Geometry: final body of the model. Coordinates: model frame, mm. A direction names the side the tool comes from. Round coordinates to 2 decimals unless told otherwise and drop trailing zeros. Loops run counter-clockwise (first coordinate to the right, second up) from the corner with the lowest first, then second, coordinate; pieces in that order, holes last. Notation, with made-up numbers: (-32.75, -6.75) - (-2.75, -6.75) arc R17 cw to (-2.75, -2.75) - close; hole circle Ø9 at (26, -14.75). An arc over 180 degrees is marked (long way). Answer in a Markdown table with one row per item. Add a question column.
from build123d import *

# Parameters (mm, degrees)
F0_R      = 18
F1_DEPTH  = 25
F2_R      = 6.5
F3_DEPTH  = 4.5
F4_R      = 1.5875
F5_DEPTH  = 9
F6_W      = 1
F6_H      = 2
F7_DEPTH  = 4.5
F8_R      = 1.5
F9_DEPTH  = 5
F10_R     = 2.5
F11_DEPTH = 4.5


# Not quite as in the source:
# - a pattern or mirror of a feature is missing from the dataset's text; its kind, count and spacing are read off the source's solid


with BuildPart() as f1:
    # F0 (on Top) → F1 (new body, symmetric)
    with BuildSketch(Plane.XY):
        Circle(F0_R)
    extrude(amount=F1_DEPTH, both=True)

    # F2 (on face) → F3 (join)
    with BuildSketch(Plane.XY.offset(25)):
        Circle(F2_R)
    extrude(amount=F3_DEPTH)

    # F4 (on face) → F5 (join)
    with BuildSketch(Plane.XY.offset(29.5)):
        Circle(F4_R)
    extrude(amount=F5_DEPTH)

    # F6 (on face) → F7 (join)
    with BuildSketch(Plane(origin=(0, 0, -25), x_dir=(1, 0, 0), z_dir=(0, 0, -1))):
        with Locations((-14.5, 0)):
            Rectangle(F6_W, F6_H)
    f7 = extrude(amount=F7_DEPTH)

    # F7_copies: F7 across plane
    add(f7.mirror(Plane(origin=(0, 0, 0), x_dir=(0, 0, 1), z_dir=(1, 0, 0))))

    # F8 (on face) → F9 (cut)
    with BuildSketch(Plane.XY.offset(25)):
        with Locations((12.5, 0)):
            Circle(F8_R)
        with Locations((-12.5, 0)):
            Circle(F8_R)
    extrude(amount=-F9_DEPTH, mode=Mode.SUBTRACT)

    # F10 (on face) → F11 (join)
    with BuildSketch(Plane(origin=(0, 0, -25), x_dir=(1, 0, 0), z_dir=(0, 0, -1))):
        Circle(F10_R)
    extrude(amount=F11_DEPTH)


solid = f1.part
1) Section A-A, the plane x = 0. Return the cut outline in (y, z), and give its area (3 significant figures).
2) Reachability of faces 4 (the cylindrical face through (-0.54, 2.44, -27.22)), 5 (the flat face through (-14, 0, -27)), 6 (the flat face through (-15, 0, -27)), 7 (the flat face through (12, 0, 20)), 8 (the flat face through (15, 0, -27)) from +Z, -Z, +X, -X, +Y, -Y: full face, straight path, thin tool, end or side. Return the list, or none.
3) Contact query for flat-ended pins moving along their axis: pin 1 Ø10 at (x, z) = (-12, -16) entering from +Y; pin 2 Ø2.5 at (x, y) = (12.5, 0) entering from +Z; pin 3 Ø1 at (y, z) = (-6.5, -0.5) entering from +X. Output: stop coordinate, or through.
4) Material intervals for line 1 along Z through (x, y) = (6, 8); line 2 along Y through (x, z) = (12.5, 22); line 3 along Y through (x, z) = (-12, 22), sorted ascending. Write a range as from..to.
5) Pull-direction query (Y, two-part tool) for faces 1 (the cylindrical face through (-5.158, -3.955, 27.218)), 2 (the flat face through (0, -8, 25)), 3 (the cylindrical face through (-14, 0, 23)); classes: pulls with the +Y half, pulls with the -Y half, needs draft (parallel to the pull), parting line crosses it, or undercut.
6) Section D-D, the plane x = 13. Return the cut outline in (y, z), and give its area (3 significant figures).
7) Section C-C, the plane y = -12.5. Return the cut outline in (x, z), and give its area (3 significant figures).
8) Section B-B, the plane z = 31.5. Return the cut outline in (x, y) (1 decimal), and give its area (3 significant figures).
Evaluation:
| question | item | result |
|---|---|---|
| 1 | outline | (-18, -25) - (-2.5, -25) - (-2.5, -29.5) - (2.5, -29.5) - (2.5, -25) - (18, -25) - (18, 25) - (6.5, 25) - (6.5, 29.5) - (1.59, 29.5) - (1.59, 38.5) - (-1.59, 38.5) - (-1.59, 29.5) - (-6.5, 29.5) - (-6.5, 25) - (-18, 25) - close |
| 1 | area | 1,910 mm² |
| 2 | face 4 | -Z |
| 2 | face 5 | -Z, +Y, -Y |
| 2 | face 6 | -Z, -X, +Y, -Y |
| 2 | face 7 | +Z |
| 2 | face 8 | -Z, +X, +Y, -Y |
| 3 | pin 1 | stops at y = 16.58 |
| 3 | pin 2 | stops at z = 20 |
| 3 | pin 3 | stops at x = 16.97 |
| 4 | line 1 | z = -25..25 |
| 4 | line 2 | y = -12.95..-1.5, 1.5..12.95 |
| 4 | line 3 | y = -13.42..-1.41, 1.41..13.42 |
| 5 | face 1 | parting line crosses it |
| 5 | face 2 | needs draft |
| 5 | face 3 | undercut |
| 6 | outline | (-12.45, -25) - (12.45, -25) - (12.45, 25) - (1.41, 25) - (1.41, 20) - (-1.41, 20) - (-1.41, 25) - (-12.45, 25) - close |
| 6 | area | 1,230 mm² |
| 7 | outline | (-12.95, -25) - (12.95, -25) - (12.95, 25) - (-12.95, 25) - close |
| 7 | area | 1,300 mm² |
| 8 | outline | circle Ø3.2 at (0, 0) |
| 8 | area | 7.92 mm² |
